Here's how the part is built. I have some questions about the finished solid (model axes, mm). Face numbers are marked on the shaded views. Coordinates: 2 decimals unless noted, no trailing zeros. Write each loop counter-clockwise with the first axis right and the second up, starting at its lowest first coordinate (ties: lowest second). Pieces come first, ordered by that corner, then holes.
(1) Imagine slicing it at B-B, the plane x = 0. List the corners of the cut face in (y, z) for me, plus the area to 3 significant figures.
(2) For pin 1 Ø1 at (y, z) = (2.5, 1.5) entering from -X, with a flat end and sliding along its axis, tell me the tip position at first contact or that it passes through.
(3) Thinking about a two-plate mould opening in X: for the marked faces 1, 2 and 3, which applies, released by +X, released by -X, zero draft, split by the parting line, or undercut?
(4) Imagine slicing it at A-A, the plane y = 2.65. List the corners of the cut face in (x, z) for me.
(5) Please list where these lines run through material, in increasing order: probe 1 along Z at (x, y) = (0, 2.1); probe 2 along Z at (x, y) = (1.75, 3.8); probe 3 along X at (y, z) = (3.8, 0).
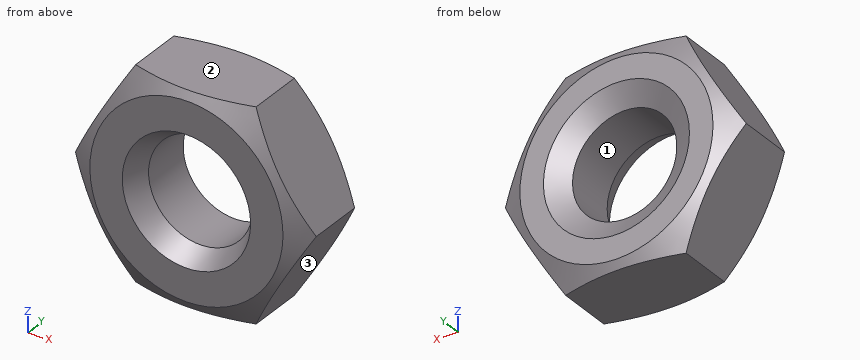
```python
from build123d import *

# Parameters (mm, degrees)
SKETCH_1_R             = 2.5
EXTRUDE_1_DEPTH        = 4
CHAMFER_1_SIZE         = 1
CHAMFER_1_SIZE2        = 0.577350269
CHAMFER_1_PART_2_SIZE  = 1
CHAMFER_1_PART_2_SIZE2 = 0.577350269


with BuildPart() as part:
    # Эскиз1 → Бобышка-Вытянуть1 (new body)
    with BuildSketch(Plane(origin=(0, 0, 0), x_dir=(1, 0, 0), z_dir=(0, 1, 0))):
        Polygon((-5.773502692, 0), (-2.886751346, -5), (2.886751346, -5), (5.773502692, 0), (2.886751346, 5), (-2.886751346, 5), align=None)
        Circle(SKETCH_1_R, mode=Mode.SUBTRACT)
    extrude(amount=EXTRUDE_1_DEPTH)

    # Фаска1
    chamfer_1_edges = [part.edges().sort_by_distance(p)[0] for p in [
        (-2.5, 0, 0),
    ]]
    chamfer_1_side = [part.faces().sort_by_distance(p)[0] for p in [
        (-2.5, 2, 0),
    ]]
    chamfer(chamfer_1_edges, length=CHAMFER_1_SIZE, length2=CHAMFER_1_SIZE2, reference=chamfer_1_side[0])

    # Фаска1 part 2
    chamfer_1_part_2_edges = [part.edges().sort_by_distance(p)[0] for p in [
        (-2.5, 4, 0),
    ]]
    chamfer_1_part_2_side = [part.faces().sort_by_distance(p)[0] for p in [
        (-4.197839453, 4, 2.423623738),
    ]]
    chamfer(chamfer_1_part_2_edges, length=CHAMFER_1_PART_2_SIZE, length2=CHAMFER_1_PART_2_SIZE2, reference=chamfer_1_part_2_side[0])

    # Эскиз2 → Вырез-Повернуть1 (revolve, cut)
    with BuildSketch(Plane(origin=(0, 0, 0), x_dir=(0, 0, -1), z_dir=(1, 0, 0))):
        Polygon((4.62815384, 0), (6.62815384, 0), (6.62815384, 1.154700538), align=None)
        Polygon((4.62815384, 4), (6.62815384, 2.845299462), (6.62815384, 4), align=None)
    revolve(axis=Axis((0, 0, 0), (0, 1, 0)), mode=Mode.SUBTRACT)


solid = part.part
```
Recorded:
1. outline: (0, -4.63) - (0.21, -5) - (3.79, -5) - (4, -4.63) - (4, -3.5) - (3.42, -2.5) - (1, -2.5) - (0, -3.08) - close; (0, 3.08) - (1, 2.5) - (3.42, 2.5) - (4, 3.5) - (4, 4.63) - (3.79, 5) - (0.21, 5) - (0, 4.63) - close
1. area: 18.7 mm2
2. pin 1: stops at x = -5.2
3. face 1: undercut
3. face 2: zero draft
3. face 3: released by +X
4. outline: (-5.77, 0) - (-2.89, -5) - (2.89, -5) - (5.77, 0) - (2.89, 5) - (-2.89, 5) - close; hole circle Ø5 at (0, 0)
5. probe 1: z = -5 to -2.5, 2.5 to 5
5. probe 2: z = -4.66 to -2.62, 2.62 to 4.66
5. probe 3: x = -4.97 to -3.15, 3.15 to 4.97
